Verification items for the finished model (mm, model axes). A direction names the side the tool comes from. Give positions to 0.01 mm unless a question says otherwise; leave off trailing zeros. Order: outer loops, then holes, each group sorted by start corner. A loop starts at its lowest first (then second) coordinate and runs counter-clockwise, first axis right, second up. Notation, with made-up numbers: (16, 54) -> (75, 54) arc R15 ccw to (75, 58) -> close; hole circle Ø8 at (83.5, 32.5). An arc over 180 degrees is marked (long way). Write each question's results on one line, items separated by ' | '. Start each with the question number.
1. Set-up check for faces 1 (the face through (102.56, 8.28, 0.51)), 2 (the face through (57, 13, 0)): record each of +Z, -Z, +X, -X, +Y, -Y from which the full face is reachable in a straight line by a thin tool's end or side.
2. Cross-section at C-C, the plane z = 0.65. Enter the section's corners in (x, y).
3. Mould release check, pull along X, two halves, no side actions. Record for faces 3 (the face through (57, 13, 1)), 4 (the face through (62.54, 8.4, 0.51)): +X half, -X half, draft (parallel to the pull), parting line (faces both ways), or undercut.
4. Cross-section at B-B, the plane y = 19.75. Enter the section's corners in (x, z).
5. Cross-section at D-D, the plane y = 15.5. Enter the section's corners in (x, z), then the cut area to 3 significant figures.
6. Cross-section at A-A, the plane x = 48. Enter the section's corners in (y, z).
7. Depth check by flat-ended pin: pin 1 Ø0.5 at (x, z) = (68, 0.5) entering from -Y. Enter the tip coordinate at first touch or a pass-through.
8. Material ranges on L1, parallel to X at y = 11, z = 0.55; L2, parallel to X at y = 18.25, z = 0.7; L3, parallel to Y at x = 47.5, z = 0.9, recorded low to high. Write a range as from..to.
from build123d import *

# Parameters (mm, degrees)
BOX_W        = 115
BOX_H        = 25.4
BOX_DEPTH    = 1
POCKET_DEPTH = 5


with BuildPart() as part:
    # Box → Box (new body)
    with BuildSketch(Plane.XY):
        with Locations((57.5, 12.7)):
            Rectangle(BOX_W, BOX_H)
    extrude(amount=BOX_DEPTH)

    # Sketch (on Face6 of BaseFeature) → Pocket (cut)
    with BuildSketch(Plane.XY.offset(1)):
        Polygon((25.040976, 4.003275), (30.040976, 12.663529), (25.040976, 21.323783), (15.040976, 21.323783), (10.040976, 12.663529), (15.040976, 4.003275), align=None)
        Polygon((50.058906, 4.004545), (55.058906, 12.664799), (50.058906, 21.325053), (40.058906, 21.325053), (35.058906, 12.664799), (40.058906, 4.004545), align=None)
        Polygon((75.076836, 4.005815), (80.076836, 12.666069), (75.076836, 21.326323), (65.076836, 21.326323), (60.076836, 12.666069), (65.076836, 4.005815), align=None)
        Polygon((100.094766, 4.007085), (105.094766, 12.667339), (100.094766, 21.327593), (90.094766, 21.327593), (85.094766, 12.667339), (90.094766, 4.007085), align=None)
    extrude(amount=-POCKET_DEPTH, mode=Mode.SUBTRACT)


solid = part.part
Results below:
1) face 1: +Z, -Z | face 2: -Z, +X, -X, +Y, -Y
2) outline: (0, 0) -> (115, 0) -> (115, 25.4) -> (0, 25.4) -> close; hole (10.04, 12.66) -> (15.04, 4) -> (25.04, 4) -> (30.04, 12.66) -> (25.04, 21.32) -> (15.04, 21.32) -> close; hole (35.06, 12.66) -> (40.06, 4) -> (50.06, 4) -> (55.06, 12.66) -> (50.06, 21.33) -> (40.06, 21.33) -> close; hole (60.08, 12.67) -> (65.08, 4.01) -> (75.08, 4.01) -> (80.08, 12.67) -> (75.08, 21.33) -> (65.08, 21.33) -> close; hole (85.09, 12.67) -> (90.09, 4.01) -> (100.09, 4.01) -> (105.09, 12.67) -> (100.09, 21.33) -> (90.09, 21.33) -> close
3) face 3: draft | face 4: undercut
4) outline: (0, 0) -> (14.13, 0) -> (14.13, 1) -> (0, 1) -> close; (25.95, 0) -> (39.15, 0) -> (39.15, 1) -> (25.95, 1) -> close; (50.97, 0) -> (64.17, 0) -> (64.17, 1) -> (50.97, 1) -> close; (75.99, 0) -> (89.18, 0) -> (89.18, 1) -> (75.99, 1) -> close; (101.01, 0) -> (115, 0) -> (115, 1) -> (101.01, 1) -> close
5) outline: (0, 0) -> (11.68, 0) -> (11.68, 1) -> (0, 1) -> close; (28.4, 0) -> (36.7, 0) -> (36.7, 1) -> (28.4, 1) -> close; (53.42, 0) -> (61.71, 0) -> (61.71, 1) -> (53.42, 1) -> close; (78.44, 0) -> (86.73, 0) -> (86.73, 1) -> (78.44, 1) -> close; (103.46, 0) -> (115, 0) -> (115, 1) -> (103.46, 1) -> close | area: 48.1 mm²
6) outline: (0, 0) -> (4, 0) -> (4, 1) -> (0, 1) -> close; (21.33, 0) -> (25.4, 0) -> (25.4, 1) -> (21.33, 1) -> close
7) pin 1: stops at y = 0
8) L1: x = 0..11, 29.08..36.02, 54.1..61.04, 79.11..86.06, 104.13..115 | L2: x = 0..13.27, 26.82..38.28, 51.83..63.3, 76.85..88.32, 101.87..115 | L3: y = 0..4, 21.33..25.4
